Solid Edge part; units mm, degrees
sketch "Sketch1" plane through (0, 0, 0) normal (0, 0, 1) x (1, 0, 0)
  line L0 (-20, 0) -> (-15, 0)
  line L1 (-15, 0) -> (-10, -5)
  line L2 (-10, -5) -> (10, -5)
  line L3 (10, -5) -> (15, 0)
  line L4 (15, 0) -> (20, 0)
  line L5 (20, 0) -> (11, -9)
  line L6 (11, -9) -> (-11, -9)
  line L7 (-11, -9) -> (-20, 0)
  dimension "D1" = 20
  dimension "D2" = 20
  dimension "D3" = 11
  dimension "D4" = 15
extrude "body_Profile_Plane1" add sketch "Sketch1" along normal mid plane 135
sketch "Sketch2" plane through (0, -5, 0) normal (0, 1, 0) x (0, 0, 1)
  circle A0 centre (27.5, 0) radius 5
  circle A1 centre (47.5, 0) radius 5
  dimension "D1" = 27.5
extrude "Protrusion1" add sketch "Sketch2" along normal up to vertex (5 mm away)
hole "Hole1" at (0, -9, 47.5) direction (0, 1, 0) diameter 3.6 end up to next counterbore diameter 6.5 counterbore depth 3.5
hole "Hole2" at (0, -9, 27.5) direction (0, 1, 0) diameter 3.6 end up to next counterbore diameter 6.5 counterbore depth 3.5
sketch "Sketch3" plane through (0, -9, 0) normal (0, -1, 0) x (0, 0, 1)
  line L0 (-67.5, 20) -> (-67.5, 14)
  line L1 (-67.5, 14) -> (-7.5, 14)
  line L2 (-7.5, 14) -> (12.5, 20)
  line L3 (12.5, 20) -> (-67.5, 20)
  dimension "D1" = 12.5
  dimension "D2" = 67.5
  dimension "D3" = 7.5
extrude "Cutout1" cut sketch "Sketch3" against normal up to vertex (9 mm away)
mirror "Mirror1" about plane through (0, 0, 0) normal (1, 0, 0) of "Cutout1"
hole "Hole3" at (0, -9, -55) direction (0, 1, 0) diameter 2.7 depth 30 tip angle 118 start chamfer 0.6 start chamfer angle 45 end chamfer 0.6 end chamfer angle 45
hole "Hole4" at (0, -9, -40) direction (0, 1, 0) diameter 2.7 depth 30 tip angle 118 start chamfer 0.6 start chamfer angle 45 end chamfer 0.6 end chamfer angle 45
sketch "Sketch4" plane through (0, -9, 0) normal (0, -1, 0) x (0, 0, 1)
  line L0 (-15, 7.5) -> (-10.6699, 0)
  line L1 (-10.6699, 0) -> (-15, -7.5)
  line L2 (-15, -7.5) -> (-12, -7.5)
  line L3 (-12, -7.5) -> (-7.6699, 0)
  line L4 (-7.6699, 0) -> (-12, 7.5)
  line L5 (-12, 7.5) -> (-15, 7.5)
  dimension "D1" = 12
extrude "design_cutout" cut sketch "Sketch4" against normal blind 0.5
pattern_linear "Pattern1" count 3 spacing 7.5 along (0, 0, 1) of "design_cutout"
properties material "Polypropylene, general purpose"
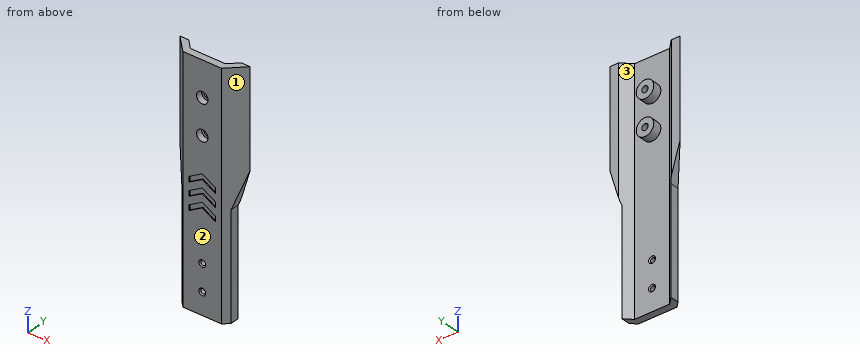
Geometry: final body of the model. Coordinates: model frame, mm. Face numbers are marked on the shaded views. Round coordinates to 2 decimals unless told otherwise and drop trailing zeros. Order: outer loops, then holes, each group sorted by start corner. A loop starts at its lowest first (then second) coordinate and runs counter-clockwise, first axis right, second up. Notation, with made-up numbers: M 42,34.25 L 48,34.25 A7 cw 48,41.25 Z; hole C 25.5,5 d4. An arc over 180 degrees is marked long. Use one line per item in the form item = value. Start each with the question number.
Q1. Cut plane A-A (z = 27.5). Return loops of the section in (x, y).
Q2. Pin query (flat end, axial travel): pin 1 Ø1 at (x, y) = (9.5, -4) entering from -Z; pin 2 Ø10.5 at (x, z) = (0, 27.5) entering from +Y; pin 3 Ø1.5 at (y, z) = (-2.5, -34.5) entering from -X; pin 4 Ø5 at (x, z) = (0, 47.5) entering from -Y. Return the tip coordinate at first contact, or that it passes through.
Q3. Mould query, pull axis X, two halves, no side actions, for the marked faces 1, 2 and 3. Classes: +X half, -X half, draft (parallel to the pull), parting line (faces both ways), or undercut.
Q4. Cut plane B-B (y = -2.75). Return loops of the section in (x, z).
Q5. Cut plane D-D (z = 10.5). Return loops of the section in (x, y).
Q6. Material intervals for line 1 (Z direction, x = 0, y = -7.7); line 2 (Y direction, x = -5, z = 20.5); line 3 (X direction, y = -2, z = 45), sorted ascending. Write a range as [from, to].
Q7. Cut plane C-C (z = -40). Return loops of the section in (x, y).
Geometry results:
q1.outline = M -20,0 L -11,-9 L -3.25,-9 L -3.25,-5.5 L -1.8,-5.5 L -1.8,0 L -5,0 L -5,-5 L -10,-5 L -15,0 Z; M 1.8,-5.5 L 3.25,-5.5 L 3.25,-9 L 11,-9 L 20,0 L 15,0 L 10,-5 L 5,-5 L 5,0 L 1.8,0 Z
q2.pin_1 = through
q2.pin_2 = 0
q2.pin_3 = -14
q2.pin_4 = -5.5
q3.face_1 = +X half
q3.face_2 = draft
q3.face_3 = undercut
q4.outline = M -17.25,3.33 L -14,-7.5 L -14,-67.5 L -12.25,-67.5 L -12.25,67.5 L -17.25,67.5 Z; C 0,27.5 d10; C 0,47.5 d10; M 12.25,-67.5 L 14,-67.5 L 14,-7.5 L 17.25,3.33 L 17.25,67.5 L 12.25,67.5 Z; hole C 0,27.5 d3.6; hole C 0,47.5 d3.6
q5.outline = M -19.4,-0.6 L -11,-9 L 11,-9 L 19.4,-0.6 L 19.4,0 L 15,0 L 10,-5 L -10,-5 L -15,0 L -19.4,0 Z
q6.line_1 = [-67.5, -56.35], [-53.65, -41.35], [-38.65, 24.25], [30.75, 44.25], [50.75, 67.5]
q6.line_2 = [-9, -5]
q6.line_3 = [-18, -13], [-4.33, 4.33], [13, 18]
q7.outline = M -14,-6 L -11,-9 L -1.95,-9 L -1.35,-8.4 L -1.35,-5.6 L -1.95,-5 L -10,-5 L -14,-1 Z; M 1.35,-8.4 L 1.95,-9 L 11,-9 L 14,-6 L 14,-1 L 10,-5 L 1.95,-5 L 1.35,-5.6 Z
